For this review, take the finished solid that the model builds, in its own axes (mm). Face numbers are marked on the shaded views. A direction names the side the tool comes from. Coordinates: 2 decimals unless noted, no trailing zeros. Loops run counter-clockwise (first coordinate to the right, second up) from the corner with the lowest first, then second, coordinate; pieces in that order, holes last. Notation, with made-up numbers: M 24,34.5 L 71,34.5 A17 cw 71,41.5 Z; hole C -29.75,9.5 d9. An arc over 180 degrees is marked long. Write item = value, one per line.
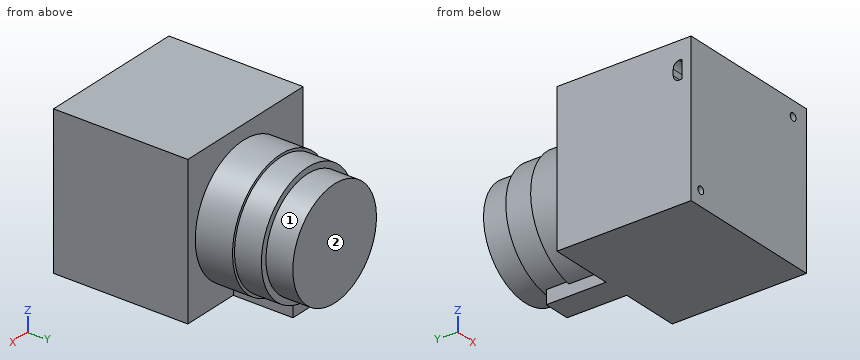
from build123d import *

# Parameters (mm, degrees)
SKETCH1_W        = 50
SKETCH1_H        = 50
EXTRUSION1_DEPTH = 45
SKETCH2_R        = 21
EXTRUSION2_DEPTH = 12.5
SKETCH3_R        = 20.13248881
EXTRUSION3_DEPTH = 9
SKETCH4_R        = 18.13248881
EXTRUSION4_DEPTH = 9
SKETCH5_W        = 9
SKETCH5_H        = 10.2
EXTRUSION5_DEPTH = 20
HOLE1_D          = 2.5
HOLE1_DEPTH      = 8
HOLE1_TIP        = 0.751075774
SKETCH8_W        = 6
SKETCH8_H        = 3
EXTRUSION6_DEPTH = 5
FILLET1_R        = 2


with BuildPart() as part:
    # Sketch1 → Extrusion1 (new body)
    with BuildSketch(Plane(origin=(0, 0, 0), x_dir=(-1, 0, 0), z_dir=(0, 1, 0))):
        with Locations((0.8, 0.8)):
            Rectangle(SKETCH1_W, SKETCH1_H)
    extrude(amount=EXTRUSION1_DEPTH)

    # Sketch2 → Extrusion2 (add)
    with BuildSketch(Plane(origin=(0, 45, 0), x_dir=(-1, 0, 0), z_dir=(0, 1, 0))):
        with Locations(Location((0, 0, 0), (0, 0, 90))):
            Circle(SKETCH2_R)
    extrude(amount=EXTRUSION2_DEPTH)

    # Sketch3 → Extrusion3 (add)
    with BuildSketch(Plane(origin=(0, 57.5, 0), x_dir=(-1, 0, 0), z_dir=(0, 1, 0))):
        with Locations(Location((0, 0, 0), (0, 0, 90))):
            Circle(SKETCH3_R)
    extrude(amount=EXTRUSION3_DEPTH)

    # Sketch4 → Extrusion4 (add)
    with BuildSketch(Plane(origin=(0, 66.5, 0), x_dir=(-1, 0, 0), z_dir=(0, 1, 0))):
        with Locations(Location((0, 0, 0), (0, 0, 90))):
            Circle(SKETCH4_R)
    extrude(amount=EXTRUSION4_DEPTH)

    # Sketch5 → Extrusion5 (add)
    with BuildSketch(Plane(origin=(0, 45, 0), x_dir=(1, 0, 0), z_dir=(0, 1, 0))):
        with Locations((0, 19.1)):
            Rectangle(SKETCH5_W, SKETCH5_H)
    extrude(amount=EXTRUSION5_DEPTH)

    # Hole1
    with Locations(Plane(origin=(0, 0, 0), x_dir=(-1, 0, 0), z_dir=(0, -1, 0))):
        with Locations((-18.420088858, -20.8), (21.579911142, 19.2)):
            Hole(HOLE1_D / 2, depth=HOLE1_DEPTH)
            with Locations((0, 0, -(HOLE1_DEPTH + HOLE1_TIP / 2))):  # 118° drill point
                Cone(0, HOLE1_D / 2, HOLE1_TIP, mode=Mode.SUBTRACT)

    # Sketch8 → Extrusion6 (cut)
    with BuildSketch(Plane.ZY.offset(25.8)):
        with Locations((16.8, 4.5)):
            Rectangle(SKETCH8_W, SKETCH8_H)
    extrude(amount=-EXTRUSION6_DEPTH, mode=Mode.SUBTRACT)

    # Fillet1
    fillet1_edges = [part.edges().sort_by_distance(p)[0] for p in [
        (-23.3, 6, 13.8),
        (-23.3, 6, 19.8),
    ]]
    fillet(fillet1_edges, radius=FILLET1_R)


solid = part.part
Q1. Add section B-B (z = 0). Write out the cut boundary in (x, y), and give its area (3 significant figures).
Solved:
outline = M -25.8,0 L 24.2,0 L 24.2,45 L 21,45 L 21,57.5 L 20.13,57.5 L 20.13,66.5 L 18.13,66.5 L 18.13,75.5 L -18.13,75.5 L -18.13,66.5 L -20.13,66.5 L -20.13,57.5 L -21,57.5 L -21,45 L -25.8,45 Z
area = 3,460 mm²
Q2. For line 1 along Y through (x, z) = (-23, 18); line 2 along Y through (x, z) = (-7, -17.5); line 3 along X through (y, z) = (2.75, 20.8), list the stretches that pass through material, from the lowest coordinate up.
Solved:
line_1 = 0 to 3, 5.99 to 45
line_2 = 0 to 66.5
line_3 = -25.8 to 17.17, 19.67 to 24.2
Q3. Machinability: for the marked faces 1 and 2, which of the approach directions +Z, -Z, +X, -X, +Y, -Y give a long, thin tool a straight path to every point of the face, cutting with its end or side? Answer none if there is none.
Solved:
face_1 = +Y
face_2 = +Z, -Z, +X, -X, +Y
Q4. For pin 1 Ø3.5 at (y, z) = (58, -23) entering from +X; pin 2 Ø6 at (y, z) = (50.5, 11) entering from +X; pin 3 Ø10 at (x, y) = (8.5, 58.5) entering from +Z, all flat-tipped, find the tip position at first contact; note any pin that passes through.
Solved:
pin_1 = 4.5
pin_2 = 19.42
pin_3 = 20.69
Q5. Add section C-C (z = -6). Write out the cut boundary in (x, y).
Solved:
outline = M -25.8,0 L 24.2,0 L 24.2,45 L 20.12,45 L 20.12,57.5 L 19.22,57.5 L 19.22,66.5 L 17.11,66.5 L 17.11,75.5 L -17.11,75.5 L -17.11,66.5 L -19.22,66.5 L -19.22,57.5 L -20.12,57.5 L -20.12,45 L -25.8,45 Z
Q6. Add section A-A (x = 0). Write out the cut boundary in (y, z).
Solved:
outline = M 0,-24.2 L 65,-24.2 L 65,-20.13 L 66.5,-20.13 L 66.5,-18.13 L 75.5,-18.13 L 75.5,18.13 L 66.5,18.13 L 66.5,20.13 L 57.5,20.13 L 57.5,21 L 45,21 L 45,25.8 L 0,25.8 Z
